For this review, take the finished solid that the model builds, in its own axes (mm). A direction names the side the tool comes from. Coordinates: 2 decimals unless noted, no trailing zeros. Write each loop counter-clockwise with the first axis right and the second up, starting at its lowest first coordinate (ties: lowest second). Pieces come first, ordered by that corner, then holes. Notation, with made-up numbers: (33, -17) - (67, -17) arc R12 cw to (67, 0) - close; hole circle Ø3 at (-20.75, 15). An arc over 180 degrees is marked (long way). Use one line per item in the form item = value. Start each with the question number.
1) For L1, parallel to Y at x = 0, z = -1.3; L2, parallel to Y at x = 45.5, z = 0.6; L3, parallel to X at y = 45, z = -1.85, list the stretches that pass through material, from the lowest coordinate up. Write a range as from..to.
2) We need section B-B (x = 37.5). Give the boundary of the cut face in (y, z), plus the area to 3 significant figures.
3) We need section C-C (y = 19). Give the boundary of the cut face in (x, z).
4) Mouldability with a two-part tool opening along X and no side actions: class faces 4 (the flat face through (3, 24, 0)), 5 (the cylindrical face through (42.5, -0.1, 1.2)), 6 (the flat face through (10.66, 29.44, -1.27)) as pulls with the +X half, pulls with the -X half, needs draft (parallel to the pull), parting line crosses it, or undercut.
5) We need section A-A (x = 44.5). Give the boundary of the cut face in (y, z).
6) Tool access review of faces 1 (the flat face through (30, 8, 1)), 2 (the flat face through (40, 0, 0)), 3 (the cylindrical face through (10.925, 9.899, -1.268)): name each direction out of +Z, -Z, +X, -X, +Y, -Y from which nothing blocks a thin tool from reaching the whole face with its end or side.
7) Insertion check: P1, Ø1.5, axis at y = 28.5, z = 1, coming from the +X side; P2, Ø2, axis at x = 33, z = 1.5, coming from the +Y side; P3, Ø5, axis at x = 36, y = 1.5, coming from the -Z side; P4, Ø8, axis at x = 1.5, y = 48, coming from the +Z side. Each pin has a flat end and moves straight along its axis. Give the tip position at first contact, or say it passes through.
Autodesk Inventor part; units mm, degrees
ref_plane "YZ Plane" through (0, 0, 0) normal (1, 0, 0) x (0, 1, 0)
ref_plane "XZ Plane" through (0, 0, 0) normal (0, 1, 0) x (-1, 0, 0)
ref_plane "XY Plane" through (0, 0, 0) normal (0, 0, 1) x (1, 0, 0)
sketch "Sketch1" plane through (0, 0, 0) normal (0, 0, 1) x (1, 0, 0)
  circle A0 centre (0, 0) radius 4
  circle A1 centre (0, 45) radius 4
  circle A2 centre (45.5, 0) radius 3
  line L0 (-7.9683, -0.7111) -> (-11.9525, 43.9333)
  arc A3 (11.9525, 43.9333) -> (-11.9525, 43.9333) centre (0, 45) ccw
  line L1 (11.9525, 43.9333) -> (9.3288, 14.5333)
  arc A4 (9.3288, 14.5333) -> (15.305, 8) centre (15.305, 14) ccw
  line L2 (15.305, 8) -> (45.5, 8)
  line L3 (45.5, -8) -> (0, -8)
  arc A5 (-7.9683, -0.7111) -> (0, -8) centre (0, 0) ccw
  arc A6 (45.5, -8) -> (45.5, 8) centre (45.5, 0) ccw
  dimension "d0" = 8
  dimension "d1" = 6
  dimension "d2" = 45
  dimension "d3" = 45.5
  dimension "d4" = 12
  dimension "d5" = 8
  dimension "d6" = 8
  dimension "d7" = 6
extrude "Extrusion1" add sketch "Sketch1" along normal mid plane 5
sketch "Sketch3" plane through (0, -8, 2.5) normal (0, -1, 0) x (1, 0, 0)
  line L0 (45.5, -5) -> (45.5, 0)
  line L1 (0, 0) -> (45.5, 0)
  line L2 (45.5, -5) -> (0, -5)
  line L3 (0, -2.5) -> (18.6731, -2.5)
  arc A0 (18.6731, -2.5) -> (21.9803, -1.25) centre (18.6731, 2.5) ccw
  arc A1 (25.2875, 0) -> (21.9803, -1.25) centre (25.2875, -5) ccw
  line L4 (45.5, -2.5) -> (26.8269, -2.5)
  arc A2 (26.8269, -2.5) -> (23.5197, -3.75) centre (26.8269, -7.5) ccw
  arc A3 (20.2125, -5) -> (23.5197, -3.75) centre (20.2125, 0) ccw
  line L5 (23.5197, -3.75) -> (21.9803, -1.25) construction
  line L6 (45.5, -2.5) -> (53.5, -2.5)
  line L7 (53.5, -2.5) -> (53.5, -5)
  line L8 (45.5, 0) -> (45.5, -5)
  line L9 (53.5, -5) -> (45.5, -5)
  line L10 (53.5, -5) -> (53.5, 0)
  line L11 (12, 0) -> (-12, 0)
  line L12 (-12, -5) -> (12, -5)
  line L13 (0, -2.5) -> (-12, -2.5)
  line L14 (-12, -5) -> (-12, 0)
  line L15 (-12, -5) -> (-12, 0)
  line L16 (-12, -5) -> (-12, 0)
  point P0 (23.5197, -0.3229)
  point P1 (22.75, -2.5)
  point P2 (22.75, -5)
  point P3 (11.9525, 0)
  point P4 (-11.9525, 0)
  point P5 (11.9525, -5)
extrude "Extrusion2" cut sketch "Sketch3" against normal through all contours L2 A3 A2 L4 L0 | L0 L6 L7 L9 | A1 A0 L3 L13 L14 L11 L1
properties part number "Elbow" material "Steel, Mild"
Determined:
q1.L1 = -8..-4, 4..41, 49..57
q1.L2 = -8..-3, 3..8
q1.L3 = -12..-4, 4..12
q2.outline = (-8, 0) - (8, 0) - (8, 2.5) - (-8, 2.5) - close
q2.area = 40.0 mm²
q3.outline = (-9.73, -2.5) - (9.73, -2.5) - (9.73, 0) - (-9.73, 0) - close
q4.face_4 = needs draft
q4.face_5 = undercut
q4.face_6 = pulls with the +X half
q5.outline = (-8, 0) - (-2.83, 0) - (-2.83, 2.5) - (-8, 2.5) - close; (2.83, 0) - (8, 0) - (8, 2.5) - (2.83, 2.5) - close
q6.face_1 = +Z, -Z, +X, +Y
q6.face_2 = -Z, +X, +Y, -Y
q6.face_3 = +Z, -Z, +X
q7.P1 = through
q7.P2 = 8
q7.P3 = 0
q7.P4 = 0
